from build123d import *

# Parameters (mm, degrees)
SKETCH1_W           = 25.4
SKETCH1_H           = 12.7
BOSS_EXTRUDE1_DEPTH = 127
SKETCH2_R           = 6.35
BOSS_EXTRUDE2_DEPTH = 25.4
BOSS_EXTRUDE3_DEPTH = 5.08


with BuildPart() as part:
    # Sketch1 → Boss-Extrude1 (new body)
    with BuildSketch(Plane.XY):
        Rectangle(SKETCH1_W, SKETCH1_H)
    extrude(amount=BOSS_EXTRUDE1_DEPTH)

    # Sketch2 → Boss-Extrude2 (add)
    with BuildSketch(Plane(origin=(0, 6.35, 0), x_dir=(1, 0, 0), z_dir=(0, 1, 0))):
        with Locations((0, -114.3)):
            Circle(SKETCH2_R)
    extrude(amount=BOSS_EXTRUDE2_DEPTH)

    # Sketch3 → Boss-Extrude3 (add)
    with BuildSketch(Plane(origin=(0, 31.75, 0), x_dir=(1, 0, 0), z_dir=(0, 1, 0))):
        with BuildLine():
            Line((5.08, -111.76), (55.88, -111.76))
            ThreePointArc((55.88, -111.76), (58.42, -114.3), (55.88, -116.84))
            Line((55.88, -116.84), (5.08, -116.84))
            ThreePointArc((5.08, -116.84), (2.54, -114.3), (5.08, -111.76))
        make_face()
        with BuildLine():
            Line((-2.54, -119.38), (-2.54, -170.18))
            ThreePointArc((-2.54, -170.18), (0, -172.72), (2.54, -170.18))
            Line((2.54, -170.18), (2.54, -119.38))
            ThreePointArc((2.54, -119.38), (0, -116.84), (-2.54, -119.38))
        make_face()
        with BuildLine():
            Line((-5.08, -111.76), (-55.88, -111.76))
            ThreePointArc((-55.88, -111.76), (-58.42, -114.3), (-55.88, -116.84))
            Line((-55.88, -116.84), (-5.08, -116.84))
            ThreePointArc((-5.08, -116.84), (-2.54, -114.3), (-5.08, -111.76))
        make_face()
        with BuildLine():
            Line((2.54, -109.22), (2.54, -58.42))
            ThreePointArc((2.54, -58.42), (0, -55.88), (-2.54, -58.42))
            Line((-2.54, -58.42), (-2.54, -109.22))
            ThreePointArc((-2.54, -109.22), (0, -111.76), (2.54, -109.22))
        make_face()
    extrude(amount=BOSS_EXTRUDE3_DEPTH)


solid = part.part
Source: CAD feature listing. Evaluate the final solid. Frame: model axes, mm. A direction names the side the tool comes from. Give positions to 0.01 mm unless a question says otherwise; leave off trailing zeros. Write each loop counter-clockwise with the first axis right and the second up, starting at its lowest first coordinate (ties: lowest second). Pieces come first, ordered by that corner, then holes. Notation, with made-up numbers: (-9.75, 14) -> (16.25, 14) arc R19 cw to (16.25, 29) -> close; hole circle Ø10 at (-24, -36.75). An arc over 180 degrees is marked (long way). Return JSON: item names as keys, results as strings. Group by question number.
1. Section C-C, the plane z = 146. Output: boundary loops of the cut face in (x, y), then the cut area to 3 significant figures.
2. Pin query (flat end, axial travel): pin 1 Ø1.5 at (y, z) = (34, 81) entering from -X; pin 2 Ø4 at (y, z) = (35.5, 71) entering from +X; pin 3 Ø6.5 at (y, z) = (2, 77.5) entering from +X. Return the tip coordinate at first contact, or that it passes through.
3. Material intervals for line 1 (X direction, y = 3, z = 36); line 2 (Z direction, x = -25, y = 32); line 3 (Y direction, x = -8, z = 71.5), sorted ascending. Write a range as from..to.
4. Mould query, pull axis Y, two halves, no side actions, for faces 1 (the face through (-2.54, 34.25, 114.36)), 2 (the face through (0, 36.83, 83)), 3 (the face through (3.414, 18.872, 108.946)), 4 (the face through (0, 31.75, 82)). Classes: +Y half, -Y half, draft (parallel to the pull), parting line (faces both ways), or undercut.
5. Access query for faces 5 (the face through (-0.06, 34.25, 172.72)), 6 (the face through (0, 31.75, 114)). Directions: +Z, -Z, +X, -X, +Y, -Y. A direction counts if a zero-diameter tool reaches every point of the face in a straight line with its end or side. Return the directions, or none.
6. Section A-A, the plane z = 73. Output: boundary loops of the cut face in (x, y), then the cut area to 3 significant figures.
7. Section D-D, the plane x = -45.5. Output: boundary loops of the cut face in (y, z), then the cut area to 3 significant figures.
8. Section B-B, the plane y = 23. Output: boundary loops of the cut face in (x, z), then the cut area to 3 significant figures.
Determined:
{
 "1": {"outline": "(-2.54, 31.75) -> (2.54, 31.75) -> (2.54, 36.83) -> (-2.54, 36.83) -> close", "area": "25.8 mm2"},
 "2": {"pin 1": "stops at x = -2.54", "pin 2": "stops at x = 2.54", "pin 3": "stops at x = 12.7"},
 "3": {"line 1": "x = -12.7..12.7", "line 2": "z = 111.76..116.84", "line 3": "y = -6.35..6.35"},
 "4": {"face 1": "draft", "face 2": "+Y half", "face 3": "undercut", "face 4": "undercut"},
 "5": {"face 5": "+Z, +Y, -Y", "face 6": "+Y"},
 "6": {"outline": "(-12.7, -6.35) -> (12.7, -6.35) -> (12.7, 6.35) -> (-12.7, 6.35) -> close; (-2.54, 31.75) -> (2.54, 31.75) -> (2.54, 36.83) -> (-2.54, 36.83) -> close", "area": "348 mm2"},
 "7": {"outline": "(31.75, 111.76) -> (36.83, 111.76) -> (36.83, 116.84) -> (31.75, 116.84) -> close", "area": "25.8 mm2"},
 "8": {"outline": "circle Ø12.7 at (0, 114.3)", "area": "127 mm2"}
}
